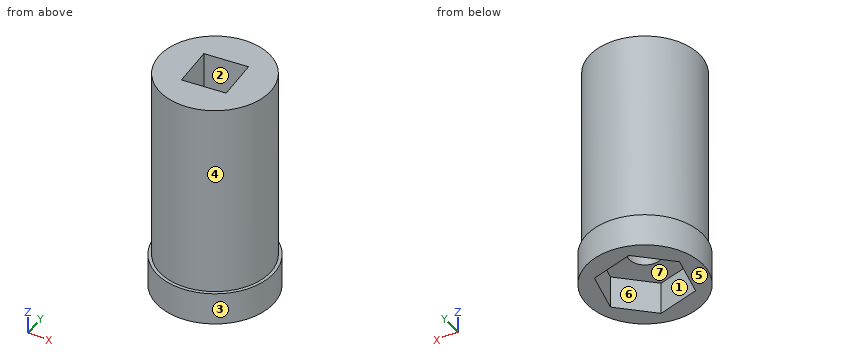
```python
from build123d import *

# Parameters (mm, degrees)
SKETCH_R      = 18.006159
PAD_DEPTH     = 10
SKETCH001_R   = 17
SKETCH001_R_2 = 4.86
PAD001_DEPTH  = 60
POCKET_DEPTH  = 20


with BuildPart() as part:
    # Sketch → Pad (new body)
    with BuildSketch(Plane.XY):
        Circle(SKETCH_R)
        Polygon((-13.231617, 4.113917), (-10.178565, -9.401958), (3.053052, -13.515875), (13.231617, -4.113917), (10.178565, 9.401958), (-3.053052, 13.515875), align=None, mode=Mode.SUBTRACT)
    extrude(amount=PAD_DEPTH)

    # Sketch001 (on Face9 of Pad) → Pad001 (join)
    with BuildSketch(Plane.XY.offset(10)):
        Circle(SKETCH001_R)
        Circle(SKETCH001_R_2, mode=Mode.SUBTRACT)
    extrude(amount=PAD001_DEPTH)

    # Sketch002 (on Face12 of Pad001) → Pocket (cut)
    with BuildSketch(Plane.XY.offset(70)):
        Polygon((-7.174122, 6.189667), (-6.189667, -7.174122), (7.174122, -6.189667), (6.189667, 7.174122), align=None)
    extrude(amount=-POCKET_DEPTH, mode=Mode.SUBTRACT)


solid = part.part
```
Build history of the part. All positions in model axes, mm. Face numbers are marked on the shaded views. A direction names the side the tool comes from. Coordinates: 2 decimals unless noted, no trailing zeros. Order: outer loops, then holes, each group sorted by start corner. A loop starts at its lowest first (then second) coordinate and runs counter-clockwise, first axis right, second up. Notation, with made-up numbers: (-40, 14.25) -> (14, 14.25) arc R13 ccw to (14, 24.25) -> close; hole circle Ø4 at (-17, 32). An arc over 180 degrees is marked (long way). Answer in a Markdown table with one row per item. Add a question column.
Q1. Wall check: line 1 along Y through (x, z) = (0, 41.5); line 2 along Z through (x, y) = (5, -7.5); line 3 along Y through (x, z) = (6, 60). Give the ranges that are in metal, low to high. Write a range as [from, to].
Q2. Band-saw the part on B-B, the plane z = 59. List the corners of the cut face in (x, y).
Q3. Band-saw the part on A-A, the plane x = 0. List the corners of the cut face in (y, z).
Q4. Band-saw the part on D-D, the plane x = -14. List the corners of the cut face in (y, z).
Q5. Mould opens along X. For the marked faces 4, 5, 6 and 7 say: +X half, -X half, draft (parallel to the pull), parting line (faces both ways), or undercut.
Q6. Drop flat-ended pins along their axis: pin 1 (10 mm diameter, centred on y = 14, z = 26.5, fed in from +X); pin 2 (10 mm diameter, centred on y = 8.5, z = 35, fed in from +X); pin 3 (6 mm diameter, centred on x = -10.5, z = 23, fed in from +Y). Give the stop position or say it passes through.
Q7. Band-saw the part on C-C, the plane y = 0. List the corners of the cut face in (x, z).
Q8. Which spindle directions (+Z, -Z, +X, -X, +Y, -Y) get a long thin tool onto all of the face, cutting with end or side? Do the marked faces 1, 2 and 3. Say none if no direction does.
Answers follow:
| question | item | result |
|---|---|---|
| 1 | line 1 | [-17, -4.86], [4.86, 17] |
| 1 | line 2 | [10, 70] |
| 1 | line 3 | [-15.91, -6.28], [7.16, 15.91] |
| 2 | outline | circle Ø34 at (0, 0); hole (-7.17, 6.19) -> (-6.19, -7.17) -> (7.17, -6.19) -> (6.19, 7.17) -> close |
| 3 | outline | (-18.01, 0) -> (-12.57, 0) -> (-12.57, 10) -> (-4.86, 10) -> (-4.86, 50) -> (-6.72, 50) -> (-6.72, 70) -> (-17, 70) -> (-17, 10) -> (-18.01, 10) -> close; (4.86, 10) -> (12.57, 10) -> (12.57, 0) -> (18.01, 0) -> (18.01, 10) -> (17, 10) -> (17, 70) -> (6.72, 70) -> (6.72, 50) -> (4.86, 50) -> close |
| 4 | outline | (-11.32, 0) -> (11.32, 0) -> (11.32, 10) -> (9.64, 10) -> (9.64, 70) -> (-9.64, 70) -> (-9.64, 10) -> (-11.32, 10) -> close |
| 5 | face 4 | parting line |
| 5 | face 5 | draft |
| 5 | face 6 | undercut |
| 5 | face 7 | undercut |
| 6 | pin 1 | x = 14.42 |
| 6 | pin 2 | x = 16.64 |
| 6 | pin 3 | y = 15.26 |
| 7 | outline | (-18.01, 0) -> (-12.3, 0) -> (-12.3, 10) -> (-4.86, 10) -> (-4.86, 50) -> (-6.72, 50) -> (-6.72, 70) -> (-17, 70) -> (-17, 10) -> (-18.01, 10) -> close; (4.86, 10) -> (12.3, 10) -> (12.3, 0) -> (18.01, 0) -> (18.01, 10) -> (17, 10) -> (17, 70) -> (6.72, 70) -> (6.72, 50) -> (4.86, 50) -> close |
| 8 | face 1 | -Z |
| 8 | face 2 | +Z |
| 8 | face 3 | +Z, -Z |
